from build123d import *

# Parameters (mm, degrees)
F0_R         = 5
F1_DEPTH     = 15
F2_W         = 2.5
F2_H         = 8
F3_DEPTH     = 25
F4_T1_DEPTH  = 8
F4_T6_ANGLE  = 323.6604372277
F4_T13_ANGLE = 323.6604372277
F4_T21_ANGLE = 323.6604372277
F4_T26_DEPTH = 15.8662197745
F4_T34_ANGLE = 323.6604372277
F4_T39_DEPTH = 15.8662197745
F4_T47_DEPTH = 15.8662197745
F4_T52_ANGLE = 323.6604372277
F4_T60_ANGLE = 323.6604372277
F4_T65_DEPTH = 15.8662197745
F5_SIZE      = 1


# Not quite as in the source:
# - a fillet or chamfer that OpenCascade refuses, or shapes differently, is made with other operations: its cross-section is extruded or revolved along the edge and cut away or added


with BuildPart() as f1:
    # F0 (on Top) → F1 (new body)
    with BuildSketch(Plane.XY):
        Circle(F0_R)
        Polygon((3.1522870356, 2.6203854256), (3.8454638641, -1.4197679401), (0.6931768285, -4.0401533656), (-3.1522870356, -2.6203854256), (-3.8454638641, 1.4197679401), (-0.6931768285, 4.0401533656), align=None, mode=Mode.SUBTRACT)
    extrude(amount=F1_DEPTH)

    # F2 (on face) → F3 (join)
    with BuildSketch(Plane(origin=(1.2295551036, 3.3302693956, 0), x_dir=(0.9381040551, -0.3463535503, 0), z_dir=(-0.3463535503, -0.9381040551, 0))):
        with Locations((0, 7.3666626269)):
            Rectangle(F2_W, F2_H)
    extrude(amount=-F3_DEPTH)

    # F4: chamfer of 5 on 4 edges, made by hand

    # F4_s2 → F4_t1 (join)
    with BuildSketch(Plane.XY.offset(3.3666626269)):
        with BuildLine():
            Line((-1.5797144045, 4.7438910612), (1.5310914666, 7.7560143709))
            Line((1.5310914666, 7.7560143709), (0.5041468464, 4.9745186659))
            ThreePointArc((0.5041468464, 4.9745186659), (-0.631305898, 4.9599851676), (-1.5797144045, 4.7438910612))
        make_face()
        with BuildLine():
            Line((4.2834359399, 2.5791813718), (3.8763516043, 6.8901304951))
            Line((3.8763516043, 6.8901304951), (2.8494069841, 4.1086347901))
            ThreePointArc((2.8494069841, 4.1086347901), (3.702995808, 3.359735413), (4.2834359399, 2.5791813718))
        make_face()
    extrude(amount=F4_T1_DEPTH)


with BuildPart() as f4_tool4:
    # F4_s5 → F4_t6 (revolve)
    with BuildSketch(Plane(origin=(0, 0, 0), x_dir=(0, 0, 1), z_dir=(0.7833222839, -0.6216157974, 0))):
        Polygon((16.3666626269, 5), (11.3666626269, 10), (11.3666626269, 5), align=None)
    revolve(axis=Axis((0, 0, 11.3666626269), (0, 0, -1)), revolution_arc=F4_T6_ANGLE)

    split(bisect_by=Plane.XY.offset(15), keep=Keep.BOTTOM)

    split(bisect_by=Plane(origin=(-1.1726300689, 0.4329419379, 0), x_dir=(0, 0, 1), z_dir=(0.9381040551, -0.3463535503, 0)), keep=Keep.TOP)

    split(bisect_by=Plane(origin=(1.1726300689, -0.4329419379, 0), x_dir=(0, 0, 1), z_dir=(-0.9381040551, 0.3463535503, 0)), keep=Keep.TOP)


with BuildPart() as f1_1:
    add(f1.part)

    # F4_t3: union F4_tool4
    add(f4_tool4.part)


with BuildPart() as f4_tool11:
    # F4_s12 → F4_t13 (revolve)
    with BuildSketch(Plane(origin=(0, 0, 0), x_dir=(0, 0, 1), z_dir=(0.7833222839, -0.6216157974, 0))):
        Polygon((-1.6333373731, 5), (3.3666626269, 10), (3.3666626269, 5), align=None)
    revolve(axis=Axis((0, 0, 3.3666626269), (0, 0, -1)), revolution_arc=F4_T13_ANGLE)

    split(bisect_by=Plane.XY, keep=Keep.TOP)

    split(bisect_by=Plane(origin=(-1.1726300689, 0.4329419379, 0), x_dir=(0, 0, 1), z_dir=(0.9381040551, -0.3463535503, 0)), keep=Keep.TOP)

    split(bisect_by=Plane(origin=(1.1726300689, -0.4329419379, 0), x_dir=(0, 0, 1), z_dir=(-0.9381040551, 0.3463535503, 0)), keep=Keep.TOP)


with BuildPart() as f1_2:
    add(f1_1.part)

    # F4_t10: union F4_tool11
    add(f4_tool11.part)


with BuildPart() as f4_tool19:
    # F4_s20 → F4_t21 (revolve)
    with BuildSketch(Plane(origin=(0, 0, 0), x_dir=(0, 0, 1), z_dir=(0.7833222839, -0.6216157974, 0))):
        Polygon((16.3666626269, 5), (11.3666626269, 10), (11.3666626269, 5), align=None)
    revolve(axis=Axis((0, 0, 11.3666626269), (0, 0, -1)), revolution_arc=F4_T21_ANGLE)

    split(bisect_by=Plane.XY.offset(15), keep=Keep.BOTTOM)

    split(bisect_by=Plane(origin=(-1.1726300689, 0.4329419379, 0), x_dir=(0, 0, 1), z_dir=(-0.9381040551, 0.3463535503, 0)), keep=Keep.TOP)


with BuildPart() as f4_tool24:
    # F4_s25 → F4_t26 (new body)
    with BuildSketch(Plane.XY.offset(19.2328824014)):
        with BuildLine():
            Line((-1.5797144045, 4.7438910612), (1.5310914666, 7.7560143709))
            Line((1.5310914666, 7.7560143709), (0.5041468464, 4.9745186659))
            ThreePointArc((0.5041468464, 4.9745186659), (-0.631305898, 4.9599851676), (-1.5797144045, 4.7438910612))
        make_face()
    extrude(amount=-F4_T26_DEPTH)

    split(bisect_by=Plane.XY.offset(15), keep=Keep.BOTTOM)

    split(bisect_by=Plane.XY.offset(11.3666626269), keep=Keep.TOP)


with BuildPart() as f4_tool19_1:
    add(f4_tool19.part)

    # F4_t29: intersect F4_tool24
    add(f4_tool24.part, mode=Mode.INTERSECT)


with BuildPart() as f1_3:
    add(f1_2.part)

    # F4_t17: union F4_tool19
    add(f4_tool19_1.part)


with BuildPart() as f4_tool32:
    # F4_s33 → F4_t34 (revolve)
    with BuildSketch(Plane(origin=(0, 0, 0), x_dir=(0, 0, 1), z_dir=(0.7833222839, -0.6216157974, 0))):
        Polygon((16.3666626269, 5), (11.3666626269, 10), (11.3666626269, 5), align=None)
    revolve(axis=Axis((0, 0, 11.3666626269), (0, 0, -1)), revolution_arc=F4_T34_ANGLE)

    split(bisect_by=Plane.XY.offset(15), keep=Keep.BOTTOM)

    split(bisect_by=Plane(origin=(1.1726300689, -0.4329419379, 0), x_dir=(0, 0, 1), z_dir=(0.9381040551, -0.3463535503, 0)), keep=Keep.TOP)


with BuildPart() as f4_tool37:
    # F4_s38 → F4_t39 (new body)
    with BuildSketch(Plane.XY.offset(19.2328824014)):
        with BuildLine():
            Line((4.2834359399, 2.5791813718), (3.8763516043, 6.8901304951))
            Line((3.8763516043, 6.8901304951), (2.8494069841, 4.1086347901))
            ThreePointArc((2.8494069841, 4.1086347901), (3.702995808, 3.359735413), (4.2834359399, 2.5791813718))
        make_face()
    extrude(amount=-F4_T39_DEPTH)

    split(bisect_by=Plane.XY.offset(15), keep=Keep.BOTTOM)

    split(bisect_by=Plane.XY.offset(11.3666626269), keep=Keep.TOP)


with BuildPart() as f4_tool32_1:
    add(f4_tool32.part)

    # F4_t42: intersect F4_tool37
    add(f4_tool37.part, mode=Mode.INTERSECT)


with BuildPart() as f1_4:
    add(f1_3.part)

    # F4_t30: union F4_tool32
    add(f4_tool32_1.part)


with BuildPart() as f4_tool45:
    # F4_s46 → F4_t47 (new body)
    with BuildSketch(Plane.XY.offset(11.3666626269)):
        with BuildLine():
            Line((-1.5797144045, 4.7438910612), (1.5310914666, 7.7560143709))
            Line((1.5310914666, 7.7560143709), (0.5041468464, 4.9745186659))
            ThreePointArc((0.5041468464, 4.9745186659), (-0.631305898, 4.9599851676), (-1.5797144045, 4.7438910612))
        make_face()
    extrude(amount=-F4_T47_DEPTH)

    split(bisect_by=Plane.XY, keep=Keep.TOP)

    split(bisect_by=Plane.XY.offset(3.3666626269), keep=Keep.BOTTOM)


with BuildPart() as f4_tool50:
    # F4_s51 → F4_t52 (revolve)
    with BuildSketch(Plane(origin=(0, 0, 0), x_dir=(0, 0, 1), z_dir=(0.7833222839, -0.6216157974, 0))):
        Polygon((-1.6333373731, 5), (3.3666626269, 10), (3.3666626269, 5), align=None)
    revolve(axis=Axis((0, 0, 3.3666626269), (0, 0, -1)), revolution_arc=F4_T52_ANGLE)

    split(bisect_by=Plane.XY, keep=Keep.TOP)

    split(bisect_by=Plane(origin=(-1.1726300689, 0.4329419379, 0), x_dir=(0, 0, 1), z_dir=(-0.9381040551, 0.3463535503, 0)), keep=Keep.TOP)


with BuildPart() as f4_tool45_1:
    add(f4_tool45.part)

    # F4_t55: intersect F4_tool50
    add(f4_tool50.part, mode=Mode.INTERSECT)


with BuildPart() as f1_5:
    add(f1_4.part)

    # F4_t43: union F4_tool45
    add(f4_tool45_1.part)


with BuildPart() as f4_tool58:
    # F4_s59 → F4_t60 (revolve)
    with BuildSketch(Plane(origin=(0, 0, 0), x_dir=(0, 0, 1), z_dir=(0.7833222839, -0.6216157974, 0))):
        Polygon((-1.6333373731, 5), (3.3666626269, 10), (3.3666626269, 5), align=None)
    revolve(axis=Axis((0, 0, 3.3666626269), (0, 0, -1)), revolution_arc=F4_T60_ANGLE)

    split(bisect_by=Plane.XY, keep=Keep.TOP)

    split(bisect_by=Plane(origin=(1.1726300689, -0.4329419379, 0), x_dir=(0, 0, 1), z_dir=(0.9381040551, -0.3463535503, 0)), keep=Keep.TOP)


with BuildPart() as f4_tool63:
    # F4_s64 → F4_t65 (new body)
    with BuildSketch(Plane.XY.offset(11.3666626269)):
        with BuildLine():
            Line((4.2834359399, 2.5791813718), (3.8763516043, 6.8901304951))
            Line((3.8763516043, 6.8901304951), (2.8494069841, 4.1086347901))
            ThreePointArc((2.8494069841, 4.1086347901), (3.702995808, 3.359735413), (4.2834359399, 2.5791813718))
        make_face()
    extrude(amount=-F4_T65_DEPTH)

    split(bisect_by=Plane.XY, keep=Keep.TOP)

    split(bisect_by=Plane.XY.offset(3.3666626269), keep=Keep.BOTTOM)


with BuildPart() as f4_tool58_1:
    add(f4_tool58.part)

    # F4_t68: intersect F4_tool63
    add(f4_tool63.part, mode=Mode.INTERSECT)


with BuildPart() as f1_6:
    add(f1_5.part)

    # F4_t56: union F4_tool58
    add(f4_tool58_1.part)

    # F5
    f5_edges = [f1_6.edges().sort_by_distance(p)[0] for p in [
        (11.061024, 26.349929, 7.366663),
        (9.888394, 26.782871, 11.366663),
        (8.715764, 27.215813, 7.366663),
        (9.888394, 26.782871, 3.366663),
    ]]
    chamfer(f5_edges, length=F5_SIZE)


solid = f1_6.part
Build history of the part. All positions in model axes, mm. A direction names the side the tool comes from. Round coordinates to 2 decimals unless told otherwise and drop trailing zeros. Write each loop counter-clockwise with the first axis right and the second up, starting at its lowest first coordinate (ties: lowest second). Pieces come first, ordered by that corner, then holes. Notation, with made-up numbers: (74, -39.75) -> (88, -39.75) arc R35 ccw to (88, -3.75) -> close; hole circle Ø5 at (65, 2.5). An arc over 180 degrees is marked (long way). Write item = value, one per line.
(1) Probe L1, parallel to Y at x = 1, z = 11.5; L2, parallel to Y at x = -1.5, z = 9.5; L3, parallel to X at y = -2.5, z = 6.5. List the from-to ranges inside material, lowest first.
Answer:
L1 = -4.9 to -3.79, 3.42 to 7.24
L2 = -4.77 to -3.23, 3.37 to 4.82
L3 = -4.33 to -3.17, 2.55 to 4.33
(2) Band-saw the part on B-B (z = 5). Give the cut face in (x, y).
Answer:
outline = (-1.58, 4.74) arc R5 ccw (long way) to (4.28, 2.58) -> (3.88, 6.89) -> (10.71, 25.41) -> (10.12, 26.7) -> (9.65, 26.87) -> (8.37, 26.28) -> (1.53, 7.76) -> close; hole (-3.85, 1.42) -> (-3.15, -2.62) -> (0.69, -4.04) -> (3.85, -1.42) -> (3.15, 2.62) -> (-0.69, 4.04) -> close
(3) Band-saw the part on C-C (x = 9.25). Give the cut face in (y, z).
Answer:
outline = (21.44, 3.37) -> (25.95, 3.37) -> (26.68, 4.05) -> (26.68, 10.68) -> (25.95, 11.37) -> (21.44, 11.37) -> close
(4) Band-saw the part on D-D (z = 2.5). Give the cut face in (x, y).
Answer:
outline = (-1.58, 4.74) arc R5 ccw (long way) to (4.28, 2.58) -> (3.88, 6.89) -> (4.31, 8.05) arc R9.13 ccw to (1.96, 8.92) -> (1.53, 7.76) -> close; hole (-3.85, 1.42) -> (-3.15, -2.62) -> (0.69, -4.04) -> (3.85, -1.42) -> (3.15, 2.62) -> (-0.69, 4.04) -> close
(5) Tool access for faces 4 (the face through (7.343, 16.281, 7.281)), 5 (the face through (2.2, 3.3, 15)), 6 (the face through (-3.5, -0.6, 7.4)): list every direction of +Z, -Z, +X, -X, +Y, -Y with a clear straight run to the whole face (end or side of a thin tool).
Answer:
face_4 = +Z, -Z, +X
face_5 = +Z, +X, -X, +Y, -Y
face_6 = +Z, -Z
(6) Band-saw the part on A-A (y = 0). Give the cut face in (x, z).
Answer:
outline = (-5, 0) -> (-3.6, 0) -> (-3.6, 15) -> (-5, 15) -> close; (3.6, 0) -> (5, 0) -> (5, 15) -> (3.6, 15) -> close
(7) Flat gauge pins, fed straight in: pin 1 (7 mm diameter, centred on x = 6.5, y = 20, fed in from +Z); pin 2 (2.5 mm diameter, centred on x = 8, y = 18, fed in from -Z); pin 3 (1.5 mm diameter, centred on y = 23.5, z = 8.5, fed in from +X); pin 4 (1 mm diameter, centred on x = 1, y = 10.5, fed in from -Z). Where does each tip first touch, or does it go through?
Answer:
pin_1 = 11.37
pin_2 = 3.37
pin_3 = 10.29
pin_4 = through
(8) Two-plate mould, pull along Y, no slides. Class faces 1 (the face through (7, 18, 11.367)), 2 (the face through (10.42, 26.05, 7.31)), 3 (the face through (-1.2, -3.34, 7.4)): pulls with the +Y half, pulls with the -Y half, needs draft (parallel to the pull), parting line crosses it, or undercut.
Answer:
face_1 = needs draft
face_2 = pulls with the +Y half
face_3 = undercut
